Geometry: final body of the model. Coordinates: model frame, mm. Face numbers are marked on the shaded views. A direction names the side the tool comes from. Give positions to 0.01 mm unless a question says otherwise; leave off trailing zeros. Write each loop counter-clockwise with the first axis right and the second up, starting at its lowest first coordinate (ties: lowest second). Pieces come first, ordered by that corner, then holes. Notation, with made-up numbers: M 48,-10 L 104,-10 A11 ccw 104,-3 Z; hole C 20,49.25 d10. An arc over 180 degrees is marked long. Use a Markdown table: item, result. Add a question column.
1) Line query: line 1 (X direction, y = -19, z = 35); line 2 (Z direction, x = -16.5, y = -19.5); line 3 (Y direction, x = 21.75, z = 20). Output: solid intervals per line, ascending.
2) Section C-C on y = -37.06. Return the cut outline in (x, z).
3) Section D-D on y = -19. Return the cut outline in (x, z), then the cut area to 3 significant figures.
4) Set-up query: the marked faces 1, 2 and 3. Return all of +Z, -Z, +X, -X, +Y, -Y with unobstructed straight access to the full face (end or side cutting, diameter ignored); none if empty.
5) Section B-B on z = 14.5. Return the cut outline in (x, y).
6) Section A-A on x = 4. Return the cut outline in (y, z), then the cut area to 3 significant figures.
7) Pin query (flat end, axial travel): pin 1 (3 mm diameter, centred on x = -7.5, z = 7.5, fed in from -Y); pin 2 (1.5 mm diameter, centred on x = -10.5, z = 36.5, fed in from +Y); pin 3 (3 mm diameter, centred on x = -10, y = -8.5, fed in from +Z); pin 4 (1.6 mm diameter, centred on x = 5, y = -19, fed in from -Z). Return the tip coordinate at first contact, or that it passes through.
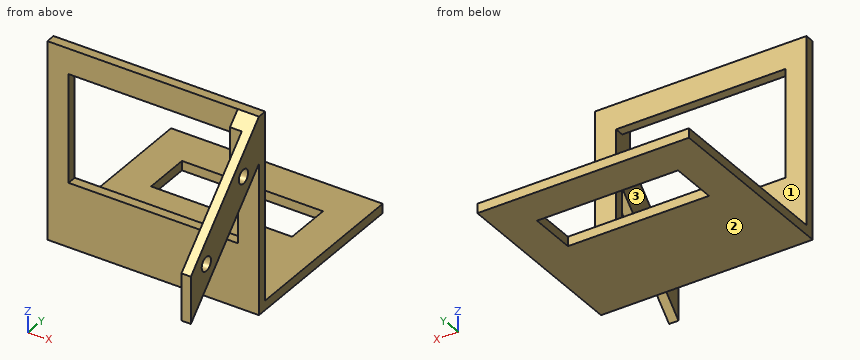
Autodesk Inventor part; units mm, degrees
ref_plane "YZ Plane" through (0, 0, 0) normal (1, 0, 0) x (0, 1, 0)
ref_plane "XZ Plane" through (0, 0, 0) normal (0, 1, 0) x (-1, 0, 0)
ref_plane "XY Plane" through (0, 0, 0) normal (0, 0, 1) x (1, 0, 0)
sketch "Boceto1" plane through (0, 0, 0) normal (0, 0, 1) x (1, 0, 0)
  line L0 (-22.5, 19.94) -> (22.5, 19.94)
  line L1 (22.5, 19.94) -> (22.5, -20.06)
  line L2 (22.5, -20.06) -> (-22.5, -20.06)
  line L3 (-22.5, -20.06) -> (-22.5, 19.94)
  line L4 (0, 19.94) -> (0, 11.94)
  line L5 (15, 12.06) -> (-15, 12.06)
  line L6 (-15, 12.06) -> (-15, 2.06)
  line L7 (-15, 2.06) -> (15, 2.06)
  line L8 (15, 2.06) -> (15, 12.06)
  point P0 (0, 0)
  dimension "d0" = 45
  dimension "d1" = 40
  dimension "d2" = 8
  dimension "d4" = 30
  dimension "d5" = 10
extrude "Extrusión1" add sketch "Boceto1" along normal blind 2
sketch "Boceto2" plane through (0, 0, 2) normal (0, 0, 1) x (1, 0, 0)
  line L0 (-22.5, 19.94) -> (-22.5, -20.06)
  line L1 (-22.5, -20.06) -> (22.5, -20.06)
  line L2 (22.5, -20.06) -> (22.5, -18.06)
  line L3 (22.5, -18.06) -> (-22.5, -18.06)
  line L4 (-22.5, -18.06) -> (-22.5, -20.06)
  point P0 (0, 0)
  dimension "d8" = 45
  dimension "d9" = 2
extrude "Extrusión2" add sketch "Boceto2" along normal blind 40
sketch "Boceto3" plane through (-22.5, -18.06, 2) normal (0, 1, 0) x (1, 0, 0)
  line L0 (22.5, -34.62) -> (4.5, -34.62)
  line L1 (4.5, -34.62) -> (4.5, -11.62)
  line L2 (4.5, -11.62) -> (40.5, -11.62)
  line L3 (40.5, -11.62) -> (40.5, -34.62)
  line L4 (40.5, -34.62) -> (22.5, -34.62)
  point P0 (22.5, 2)
  dimension "d15" = 23
  dimension "d16" = 36
extrude "Extrusión3" cut sketch "Boceto3" against normal blind 2
sketch "Boceto4" plane through (22.5, -20.06, 0) normal (1, 0, 0) x (0, 0, -1)
  line L0 (-20, -22) -> (-42, 0)
  line L1 (-20, -22) -> (-10, -22)
  line L2 (-10, -22) -> (-32, 0)
  line L3 (-42, 0) -> (-32, 0)
  point P0 (0, 20.06)
  dimension "d38" = 10
extrude "Extrusión4" add sketch "Boceto4" against normal blind 2
sketch "Boceto6" plane through (22.5, 19.94, 2) normal (1, 0, 0) x (0, 0, -1)
  line L0 (-40, -40) -> (-40, -45)
  circle A0 centre (-30, -45) radius 1.5
  circle A1 centre (-18, -57) radius 1.5
  point P0 (2, -19.94)
  dimension "d31" = 5
extrude "Extrusión6" cut sketch "Boceto6" against normal blind 2
sketch "Boceto7" plane through (0, 0, 42) normal (0, 0, 1) x (1, 0, 0)
  line L0 (-22.5, -20.06) -> (20.5, -20.06)
  line L1 (20.5, -20.06) -> (18, -20.06)
  line L2 (18, -20.06) -> (18, -22.56)
  line L3 (18, -22.56) -> (20.5, -22.56)
  line L4 (20.5, -20.06) -> (20.5, -42.06)
  line L5 (20.5, -20.06) -> (20.5, -22.56)
  point P0 (0, 0)
  dimension "d39" = 2.5
  dimension "d40" = 2.5
extrude "Extrusión7" add sketch "Boceto7" against normal blind 12.5
sketch "Boceto9" plane through (20.5, -22.56, 42) normal (1, 0, 0) x (0, 0, -1)
  line L0 (22, -19.5) -> (2.5, 0)
  line L1 (0, 2.5) -> (0, 0)
  line L2 (2.5, 0) -> (0, 0)
  line L3 (0, 0) -> (0, 2.5)
  line L4 (0, 2.5) -> (2.5, 0)
  line L5 (0, 2.5) -> (22, -19.5)
  point P0 (42, 22.56)
extrude "Extrusión8" cut sketch "Boceto9" against normal blind 12
sketch "Boceto10" plane through (20.5, -22.56, 29.5) normal (1, 0, 0) x (0, 0, -1)
  line L0 (-2.5, 2.5) -> (0, 2.5)
  line L1 (0, 0) -> (0, 2.5)
  line L2 (-2.5, 2.5) -> (0, 0)
  line L3 (0, 2.5) -> (-2.5, 2.5)
  line L4 (-2.5, 2.5) -> (0, 0)
  point P0 (29.5, 22.56)
extrude "Extrusión9" cut sketch "Boceto10" against normal blind 12
properties part number "_3DPrint"
Found:
| question | item | result |
|---|---|---|
| 1 | line 1 | -22.5 to -18, 18 to 22.5 |
| 1 | line 2 | 0 to 13.62, 36.62 to 42 |
| 1 | line 3 | -42.06 to -38.56, -35.56 to -32.06, -20.06 to -18.06 |
| 2 | outline | M 20.5,15 L 22.5,15 L 22.5,18.5 L 20.5,18.5 Z; M 20.5,21.5 L 22.5,21.5 L 22.5,25 L 20.5,25 Z |
| 3 | outline | M -22.5,0 L 22.5,0 L 22.5,42 L -22.5,42 Z; hole M -18,13.62 L 18,13.62 L 18,36.62 L -18,36.62 Z |
| 3 | area | 1,060 mm² |
| 4 | face 1 | +Z, +X, -X, +Y |
| 4 | face 2 | -Z, +X, -X, +Y, -Y |
| 4 | face 3 | +Z, -Z, -X, -Y |
| 5 | outline | M -22.5,-20.06 L -18,-20.06 L -18,-18.06 L -22.5,-18.06 Z; M 18,-20.06 L 22.5,-20.06 L 22.5,-18.06 L 18,-18.06 Z; M 20.5,-42.06 L 22.5,-42.06 L 22.5,-37.56 L 20.5,-37.56 Z |
| 6 | outline | M -20.06,0 L 2.06,0 L 2.06,2 L -18.06,2 L -18.06,13.62 L -20.06,13.62 Z; M -20.06,36.62 L -18.06,36.62 L -18.06,42 L -20.06,42 Z; M 12.06,0 L 19.94,0 L 19.94,2 L 12.06,2 Z |
| 6 | area | 94.0 mm² |
| 7 | pin 1 | y = -20.06 |
| 7 | pin 2 | y = -18.06 |
| 7 | pin 3 | z = 2 |
| 7 | pin 4 | z = 0 |
